Verification items for this drawing (mm, ordinates from the low corner). Round coordinates to 2 decimals unless told otherwise and drop trailing zeros. Order: outer loops, then holes, each group sorted by start corner. A loop starts at its lowest first (then second) coordinate and runs counter-clockwise, first axis right, second up.
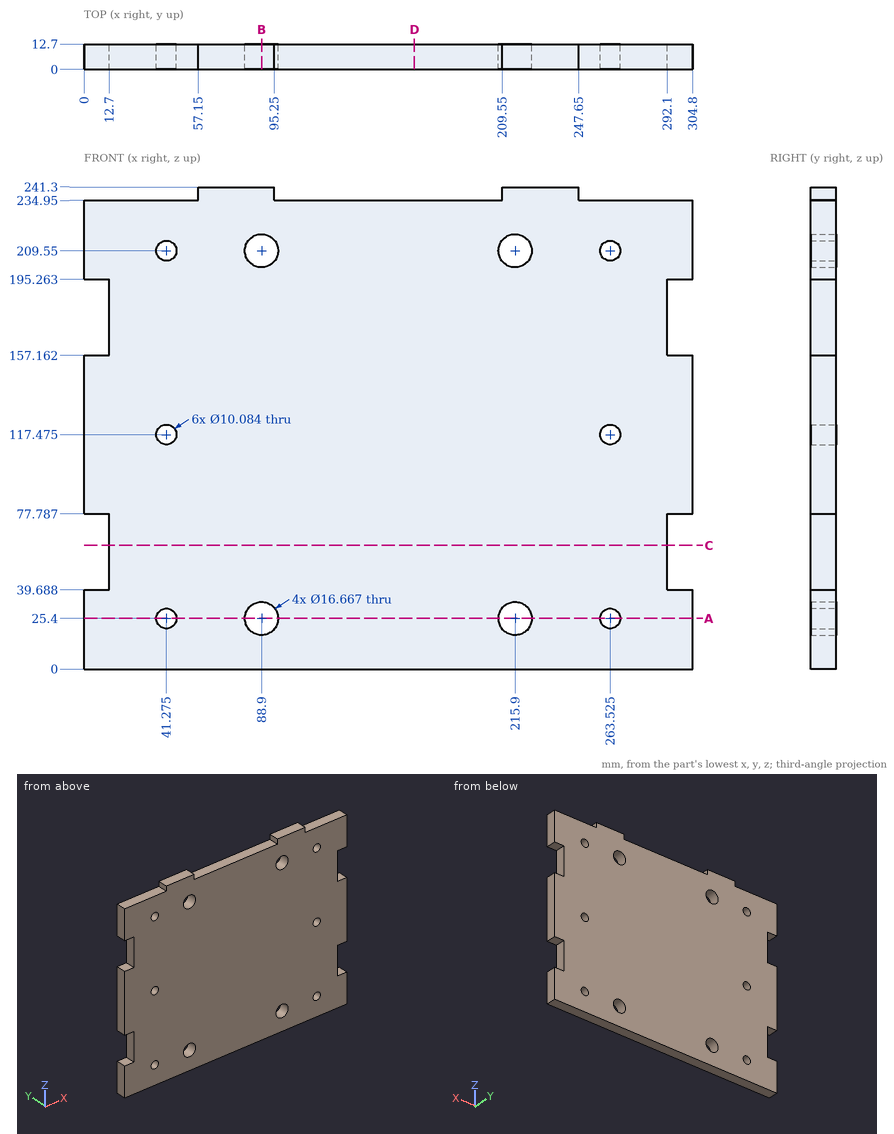
Item 1: Sectioned sample at C-C (z = 62). Record the cut outline in (x, y), and give its area (3 significant figures).
Answer:
outline: (12.7, 0) - (292.1, 0) - (292.1, 12.7) - (12.7, 12.7) - close
area: 3,550 mm2
Item 2: Sectioned sample at B-B (x = 88.9). Record the cut outline in (y, z), and give its area (3 significant figures).
Answer:
outline: (0, 0) - (12.7, 0) - (12.7, 17.07) - (0, 17.07) - close; (0, 33.73) - (12.7, 33.73) - (12.7, 201.22) - (0, 201.22) - close; (0, 217.88) - (12.7, 217.88) - (12.7, 241.3) - (0, 241.3) - close
area: 2,640 mm2
Item 3: Sectioned sample at A-A (z = 25.4). Record the cut outline in (x, y), and give its area (3 significant figures).
Answer:
outline: (0, 0) - (36.23, 0) - (36.23, 12.7) - (0, 12.7) - close; (46.32, 0) - (80.57, 0) - (80.57, 12.7) - (46.32, 12.7) - close; (97.23, 0) - (207.57, 0) - (207.57, 12.7) - (97.23, 12.7) - close; (224.23, 0) - (258.48, 0) - (258.48, 12.7) - (224.23, 12.7) - close; (268.57, 0) - (304.8, 0) - (304.8, 12.7) - (268.57, 12.7) - close
area: 3,190 mm2
Item 4: Go/stop test with flat-tipped pins: P1, Ø2, axis at y = 10.5, z = 42, coming from the +X side; P2, Ø4, axis at x = 132, y = 7, coming from the +Z side; P3, Ø13.5, axis at x = 88.9, z = 209.55, coming from the +Y side; P4, Ø1.9, axis at y = 4, z = 239, coming from the -X side. Record where each tip stops, or that it passes through.
Answer:
P1: stops at x = 292.1
P2: stops at z = 234.95
P3: passes through
P4: stops at x = 57.15
Item 5: Sectioned sample at D-D (x = 165.5). Record the cut outline in (y, z).
Answer:
outline: (0, 0) - (12.7, 0) - (12.7, 234.95) - (0, 234.95) - close
Item 6: Scan lines: line 1 along Z through (x, y) = (213, 5.5); line 2 along X through (y, z) = (8, 21) (1 decimal); line 3 along Z through (x, y) = (87, 4.25) (1 decimal). Record each from-to range of solid material in increasing order.
Answer:
line 1: z = 0 to 17.59, 33.21 to 201.74, 217.36 to 241.3
line 2: x = 0 to 38.8, 43.7 to 81.8, 96 to 208.8, 223 to 261.1, 266 to 304.8
line 3: z = 0 to 17.3, 33.5 to 201.4, 217.7 to 241.3
